Geometry check sheet. Reference: the model listing, model coordinates, mm. A direction names the side the tool comes from. Round coordinates to 2 decimals unless told otherwise and drop trailing zeros. Write each loop counter-clockwise with the first axis right and the second up, starting at its lowest first coordinate (ties: lowest second). Pieces come first, ordered by that corner, then holes.
Item 1: Depth check by flat-ended pin: P1, Ø1, axis at y = 10, z = -8, coming from the -X side; P2, Ø2.5, axis at x = 0, z = -9.5, coming from the +Y side; P3, Ø1.8, axis at x = 9.5, z = 0, coming from the -Y side. Enter the tip coordinate at first touch or a pass-through.
Item 2: Cross-section at B-B (z = -7). Enter the section's corners in (x, y).
Item 3: Draft check along Z on faces 4 (the face through (-5.2, 2, -0.2)), 5 (the face through (0, 1, -11)), 6 (the face through (1.05, 3.1, 4.75)). Enter one of: pulls with the +Z half, pulls with the -Z half, needs draft (parallel to the pull), parting line crosses it, or undercut.
Item 4: Cross-section at D-D (z = 4). Enter the section's corners in (x, y), then the cut area to 3 significant figures.
Item 5: Cross-section at C-C (x = -7). Enter the section's corners in (y, z).
Item 6: Scan lines: probe 1 along Z at (x, y) = (0, 1.25); probe 2 along Y at (x, z) = (-9.5, 5); probe 3 along Y at (x, z) = (6.5, 14). Record each from-to range of solid material in increasing order.
Item 7: Cross-section at A-A (x = 0). Enter the section's corners in (y, z).
Item 8: Access from +Z, -Z, +X, -X, +Y, -Y to the whole of each face (thin tool, end or side, straight path). Record for faces 1 (the face through (-3.9, 4.162, 3.5)), 2 (the face through (2.5, 27.1, 0.1)), 3 (the face through (0, 1, 8)).
from build123d import *

# Parameters (mm, degrees)
SKETCH4_R           = 2.5
BOSS_EXTRUDE1_DEPTH = 15
SKETCH5_R           = 1.5
CUT_EXTRUDE3_DEPTH  = 4


with BuildPart() as part:
    # Sketch3 → Revolve1 (revolve)
    with BuildSketch(Plane.XY, mode=Mode.PRIVATE) as revolve1_sk:
        Polygon((0, 0), (12, 0), (12, 2), (4.864864865, 2), (4.864864865, 4.162162162), (16.7, 4.162162162), (16.7, 19.7), (0, 19.7), align=None)
    revolve(revolve1_sk.sketch.rotate(Axis((0, 19.7, 0), (0, -1, 0)), 180), axis=Axis((0, 19.7, 0), (0, -1, 0)))

    # Sketch4 → Boss-Extrude1 (add)
    with BuildSketch(Plane(origin=(0, 19.7, 0), x_dir=(1, 0, 0), z_dir=(0, 1, 0))):
        with Locations(Location((0, 0, 0), (0, 0, 180))):
            Circle(SKETCH4_R)
    extrude(amount=BOSS_EXTRUDE1_DEPTH)

    # Sketch5 → Cut-Extrude3 (cut)
    with BuildSketch(Plane.XZ):
        with Locations((9.5, 0)):
            Circle(SKETCH5_R)
        with Locations((0, -9.5)):
            Circle(SKETCH5_R)
        with Locations((-9.5, 0)):
            Circle(SKETCH5_R)
        with Locations((0, 9.5)):
            Circle(SKETCH5_R)
    extrude(amount=-CUT_EXTRUDE3_DEPTH, mode=Mode.SUBTRACT)


solid = part.part
Resolved:
1. P1: stops at x = -14.92
1. P2: stops at y = 19.7
1. P3: stops at y = 4.16
2. outline: (-15.16, 4.16) - (15.16, 4.16) - (15.16, 19.7) - (-15.16, 19.7) - close; (-9.75, 0) - (9.75, 0) - (9.75, 2) - (-9.75, 2) - close
3. face 4: needs draft
3. face 5: undercut
3. face 6: parting line crosses it
4. outline: (-16.21, 4.16) - (-2.77, 4.16) - (-2.77, 2) - (-11.31, 2) - (-11.31, 0) - (11.31, 0) - (11.31, 2) - (2.77, 2) - (2.77, 4.16) - (16.21, 4.16) - (16.21, 19.7) - (-16.21, 19.7) - close
4. area: 561 mm2
5. outline: (0, -9.75) - (2, -9.75) - (2, 9.75) - (0, 9.75) - close; (4.16, -15.16) - (19.7, -15.16) - (19.7, 15.16) - (4.16, 15.16) - close
6. probe 1: z = -12 to -11, -8 to 8, 11 to 12
6. probe 2: y = 0 to 2, 4.16 to 19.7
6. probe 3: y = 4.16 to 19.7
7. outline: (0, -12) - (2, -12) - (2, -11) - (0, -11) - close; (0, -8) - (2, -8) - (2, -4.86) - (4.16, -4.86) - (4.16, -16.7) - (19.7, -16.7) - (19.7, -2.5) - (34.7, -2.5) - (34.7, 2.5) - (19.7, 2.5) - (19.7, 16.7) - (4.16, 16.7) - (4.16, 4.86) - (2, 4.86) - (2, 8) - (0, 8) - close; (0, 11) - (2, 11) - (2, 12) - (0, 12) - close
8. face 1: none
8. face 2: +Y
8. face 3: -Y
